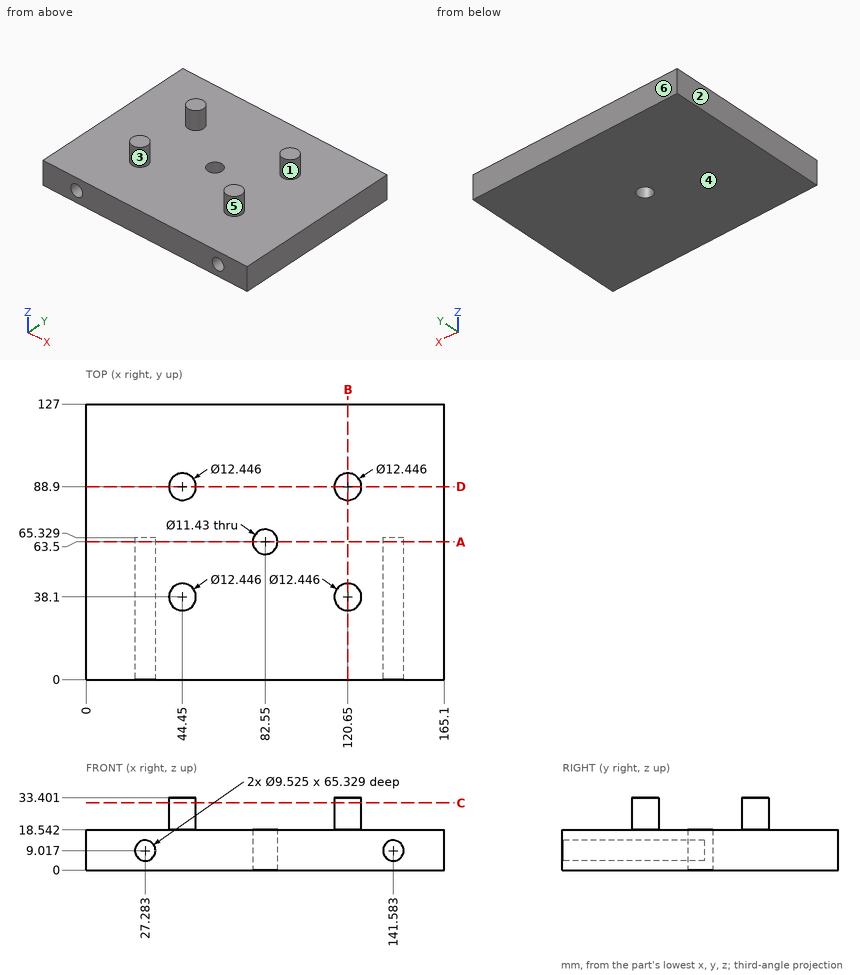
For this review, use the dimensioned drawing (mm, ordinates from the lowest corner) and the shaded views. A direction names the side the tool comes from. Give positions to 0.01 mm unless a question says otherwise; leave off trailing zeros. Write each loop counter-clockwise with the first axis right and the second up, starting at its lowest first coordinate (ties: lowest second). Pieces come first, ordered by that corner, then holes.
(1) To check wall thickness, follow L1, parallel to Z at x = 110.5, y = 79; L2, parallel to X at y = 67, z = 3.5; L3, parallel to X at y = 91, z = 22. State the ranges of each line that lie inside material, in increasing order.
(2) Consider section A-A, the plane y = 63.5. Give the boundary of the cut face in (x, z) (1 decimal), and give its area (3 significant figures).
(3) Consider section D-D, the plane y = 88.9. Give the boundary of the cut face in (x, z), and give its area (3 significant figures).
(4) Tool access review of the marked faces 5 and 6: name each direction out of +Z, -Z, +X, -X, +Y, -Y from which nothing blocks a thin tool from reaching the whole face with its end or side.
(5) The part is to be moulded in two halves that separate along X. For the marked faces 1, 2, 3 and 4, say which applies: released by +X, released by -X, zero draft, split by the parting line, or undercut.
(6) Consider section B-B, the plane x = 120.65. Give the boundary of the cut face in (y, z), and give its area (3 significant figures).
(7) For P1, Ø2, axis at x = 62, y = 58, coming from the +Z side; P2, Ø5.5, axis at x = 27.28, z = 9.02, coming from the -Y side; P3, Ø6, axis at y = 37, z = 22, coming from the -X side; P4, Ø7, axis at x = 82.55, y = 63.5, coming from the -Z side, all flat-tipped, find the tip position at first contact; note any pin that passes through.
(8) Consider section C-C, the plane z = 31. Give the boundary of the cut face in (x, y), and give its area (3 significant figures).
Returned:
1. L1: z = 0 to 18.54
1. L2: x = 0 to 78.03, 87.07 to 165.1
1. L3: x = 38.59 to 50.31, 114.79 to 126.51
2. outline: (0, 0) - (76.8, 0) - (76.8, 18.5) - (0, 18.5) - close; (88.3, 0) - (165.1, 0) - (165.1, 18.5) - (88.3, 18.5) - close; hole circle Ø9.5 at (27.3, 9); hole circle Ø9.5 at (141.6, 9)
2. area: 2,710 mm2
3. outline: (0, 0) - (165.1, 0) - (165.1, 18.54) - (126.87, 18.54) - (126.87, 33.4) - (114.43, 33.4) - (114.43, 18.54) - (50.67, 18.54) - (50.67, 33.4) - (38.23, 33.4) - (38.23, 18.54) - (0, 18.54) - close
3. area: 3,430 mm2
4. face 5: +Z
4. face 6: +Z, -Z, +X, -X, +Y
5. face 1: undercut
5. face 2: released by -X
5. face 3: undercut
5. face 4: zero draft
6. outline: (0, 0) - (127, 0) - (127, 18.54) - (95.12, 18.54) - (95.12, 33.4) - (82.68, 33.4) - (82.68, 18.54) - (44.32, 18.54) - (44.32, 33.4) - (31.88, 33.4) - (31.88, 18.54) - (0, 18.54) - close
6. area: 2,720 mm2
7. P1: stops at z = 18.54
7. P2: stops at y = 65.33
7. P3: stops at x = 38.23
7. P4: passes through
8. outline: circle Ø12.45 at (44.45, 38.1); circle Ø12.45 at (44.45, 88.9); circle Ø12.45 at (120.65, 38.1); circle Ø12.45 at (120.65, 88.9)
8. area: 487 mm2
